Input: part model. Units: mm. Frame: model coordinates. Coordinates: 2 decimals unless noted, no trailing zeros. Loops run counter-clockwise (first coordinate to the right, second up) from the corner with the lowest first, then second, coordinate; pieces in that order, holes last.
```python
from build123d import *

# Parameters (mm, degrees)
CYLINDER_R     = 16.5
CYLINDER_DEPTH = 13


with BuildPart() as cilindro:
    # Cylinder → Cylinder (new body)
    with BuildSketch(Plane.XY):
        Circle(CYLINDER_R)
    extrude(amount=CYLINDER_DEPTH)


with BuildPart() as fusion:
    # Cone → Cone (revolve)
    with BuildSketch(Plane(origin=(0, 0, -5), x_dir=(1, 0, 0), z_dir=(0, -1, 0))):
        Polygon((0, 0), (3.5, 0), (16.5, 5), (0, 5), align=None)
    revolve(axis=Axis((0, 0, -5), (0, 0, 1)))

    # Fusion: union Cilindro
    add(cilindro.part)


solid = fusion.part
```
Item 1: Section query D-D (z = 2). Output: boundary loops of the cut face in (x, y), then the cut area to 3 significant figures.
Result:
outline: circle Ø33 at (0, 0)
area: 855 mm2
Item 2: Contact query for flat-ended pins moving along their axis: P1, Ø5, axis at x = -4.5, z = 3, coming from the +Y side; P2, Ø2, axis at x = 3, y = -4.5, coming from the -Z side; P3, Ø5, axis at y = 4, z = 0, coming from the -X side. Output: stop coordinate, or through.
Result:
P1: stops at y = 16.38
P2: stops at z = -4.65
P3: stops at x = -16.43
Item 3: Section query C-C (z = -2.5). Output: boundary loops of the cut face in (x, y).
Result:
outline: circle Ø20 at (0, 0)
Item 4: Section query A-A (y = 0). Output: boundary loops of the cut face in (x, z), then the cut area to 3 significant figures.
Result:
outline: (-16.5, 0) - (-3.5, -5) - (3.5, -5) - (16.5, 0) - (16.5, 13) - (-16.5, 13) - close
area: 529 mm2
Item 5: Line query: L1, parallel to Y at x = 1, z = 2.5; L2, parallel to Y at x = -5.5, z = 3.5; L3, parallel to Z at x = 7, y = 13. Output: solid intervals per line, ascending.
Result:
L1: y = -16.47 to 16.47
L2: y = -15.56 to 15.56
L3: z = -0.67 to 13
